Here's how the part is built. I have some questions about the finished solid (model axes, mm). Round coordinates to 2 decimals unless told otherwise and drop trailing zeros. Write each loop counter-clockwise with the first axis right and the second up, starting at its lowest first coordinate (ties: lowest second). Pieces come first, ordered by that corner, then holes. Notation, with made-up numbers: (35.25, 66.5) - (55.25, 66.5) arc R14 ccw to (55.25, 90.5) - close; hole circle Ø4 at (-23, -23). An arc over 180 degrees is marked (long way). One line per question, with ' | ' between items. Start each with the question number.
(1) If I drill on L1, parallel to X at y = 10, z = 10.75; L2, parallel to Y at x = -10, z = 49; L3, parallel to Y at x = -11, z = 9, over which ranges is the centre line in solid material (lowest first)?
(2) Will these pins go through, and if not, where does the flat tip stop? pin 1 (3 mm diameter, centred on x = -10, y = 10, fed in from -Z); pin 2 (1.5 mm diameter, centred on y = 4, z = 13, fed in from -X).
(3) Imagine slicing it at C-C (z = 30). Write out the boundary of the cut face in (x, y).
(4) Imagine slicing it at B-B (x = -10). Write out the boundary of the cut face in (y, z).
(5) Imagine slicing it at A-A (y = 10). Write out the boundary of the cut face in (x, z).
(6) Imagine slicing it at D-D (z = 10). Write out the boundary of the cut face in (x, y), plus the area to 3 significant figures.
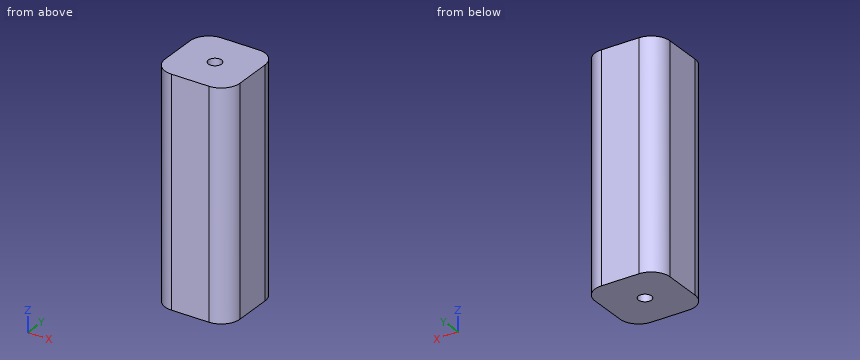
from build123d import *

# Parameters (mm, degrees)
ESQUISSE1_W             = 20
ESQUISSE1_H             = 20
BOSS_EXTRU_1_DEPTH      = 60
ESQUISSE2_R             = 1.75
ENL_V_MAT_EXTRU_1_DEPTH = 15
ENL_V_START             = -15
ESQUISSE3_R             = 1.75
ENL_V_MAT_EXTRU_2_DEPTH = 15
CONG_1_R                = 5


with BuildPart() as part:
    # Esquisse1 → Boss.-Extru.1 (new body)
    with BuildSketch(Plane.XY):
        with Locations((-10, 10)):
            Rectangle(ESQUISSE1_W, ESQUISSE1_H)
    extrude(amount=BOSS_EXTRU_1_DEPTH)

    # Esquisse2 → Enlèv. mat.-Extru.1 (cut)
    with BuildSketch(Plane.XY.offset(60)):
        with Locations((-10, 10)):
            Circle(ESQUISSE2_R)
    extrude(amount=-ENL_V_MAT_EXTRU_1_DEPTH, mode=Mode.SUBTRACT)

    # Esquisse3 → Enlèv. mat.-Extru.2 (cut)
    with BuildSketch(Plane(origin=(0, 0, 0), x_dir=(-1, 0, 0), z_dir=(0, 0, -1)).offset(ENL_V_START)):
        with Locations(Location((10, 10, 0), (0, 0, 180))):
            Circle(ESQUISSE3_R)
    extrude(amount=ENL_V_MAT_EXTRU_2_DEPTH, mode=Mode.SUBTRACT)

    # Congé1
    cong_1_edges = [part.edges().sort_by_distance(p)[0] for p in [
        (0, 0, 30),
        (-20, 0, 30),
        (-20, 20, 30),
        (0, 20, 30),
    ]]
    fillet(cong_1_edges, radius=CONG_1_R)


solid = part.part
Check sheet entries:
1) L1: -20 to -11.75, -8.25 to 0 | L2: 0 to 8.25, 11.75 to 20 | L3: 0 to 8.56, 11.44 to 20
2) pin 1: z = 15 | pin 2: x = -19.99
3) outline: (-20, 5) arc R5 ccw to (-15, 0) - (-5, 0) arc R5 ccw to (0, 5) - (0, 15) arc R5 ccw to (-5, 20) - (-15, 20) arc R5 ccw to (-20, 15) - close
4) outline: (0, 0) - (8.25, 0) - (8.25, 15) - (11.75, 15) - (11.75, 0) - (20, 0) - (20, 60) - (11.75, 60) - (11.75, 45) - (8.25, 45) - (8.25, 60) - (0, 60) - close
5) outline: (-20, 0) - (-11.75, 0) - (-11.75, 15) - (-8.25, 15) - (-8.25, 0) - (0, 0) - (0, 60) - (-8.25, 60) - (-8.25, 45) - (-11.75, 45) - (-11.75, 60) - (-20, 60) - close
6) outline: (-20, 5) arc R5 ccw to (-15, 0) - (-5, 0) arc R5 ccw to (0, 5) - (0, 15) arc R5 ccw to (-5, 20) - (-15, 20) arc R5 ccw to (-20, 15) - close; hole circle Ø3.5 at (-10, 10) | area: 369 mm^2
